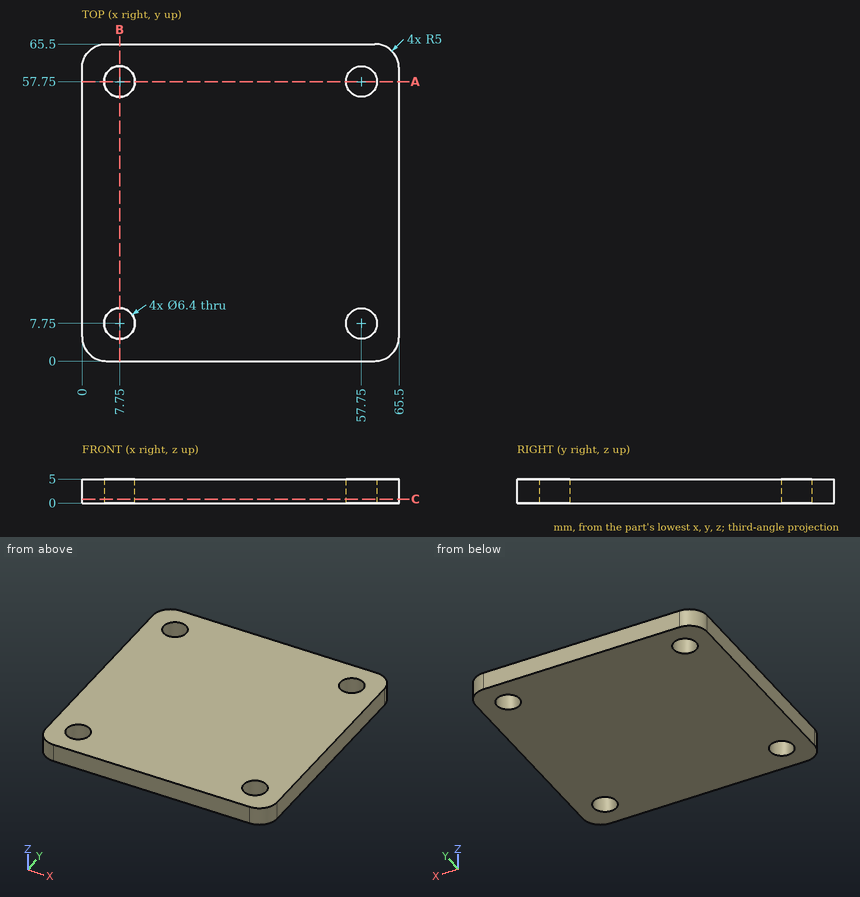
Print and shaded views of the part. All mm, measured from the part's lowest x, y and z. Give positions to 0.01 mm unless a question says otherwise; leave off trailing zeros. Loops run counter-clockwise (first coordinate to the right, second up) from the corner with the lowest first, then second, coordinate; pieces in that order, holes last. Notation, with made-up numbers: (-31.75, 33.5) - (-16.75, 33.5) arc R27 ccw to (-16.75, 67.5) - close; hole circle Ø10 at (82.25, -20.5). An arc over 180 degrees is marked (long way). One line per item, written item: value. Start each with the question number.
1. Probe L1, parallel to Y at x = 57.75, z = 3.75; L2, parallel to X at y = 55.5, z = 2.8; L3, parallel to X at y = 61.5, z = 4.75. List the from-to ranges inside material, lowest first. Write a range as from..to.
2. Slice it at C-C (z = 0.85). List the corners of the cut face in (x, y).
3. Slice it at A-A (y = 57.75). List the corners of the cut face in (x, z).
4. Pin check, flat tip, straight feed: pin 1 (5 mm diameter, centred on x = 7.75, y = 57.75, fed in from +Z). Stop position of the tip, or through.
Solution:
1. L1: y = 0..4.55, 10.95..54.55, 60.95..65.5
1. L2: x = 0..5.47, 10.03..55.47, 60.03..65.5
1. L3: x = 0.1..65.4
2. outline: (0, 5) arc R5 ccw to (5, 0) - (60.5, 0) arc R5 ccw to (65.5, 5) - (65.5, 60.5) arc R5 ccw to (60.5, 65.5) - (5, 65.5) arc R5 ccw to (0, 60.5) - close; hole circle Ø6.4 at (7.75, 7.75); hole circle Ø6.4 at (7.75, 57.75); hole circle Ø6.4 at (57.75, 7.75); hole circle Ø6.4 at (57.75, 57.75)
3. outline: (0, 0) - (4.55, 0) - (4.55, 5) - (0, 5) - close; (10.95, 0) - (54.55, 0) - (54.55, 5) - (10.95, 5) - close; (60.95, 0) - (65.5, 0) - (65.5, 5) - (60.95, 5) - close
4. pin 1: passes through
